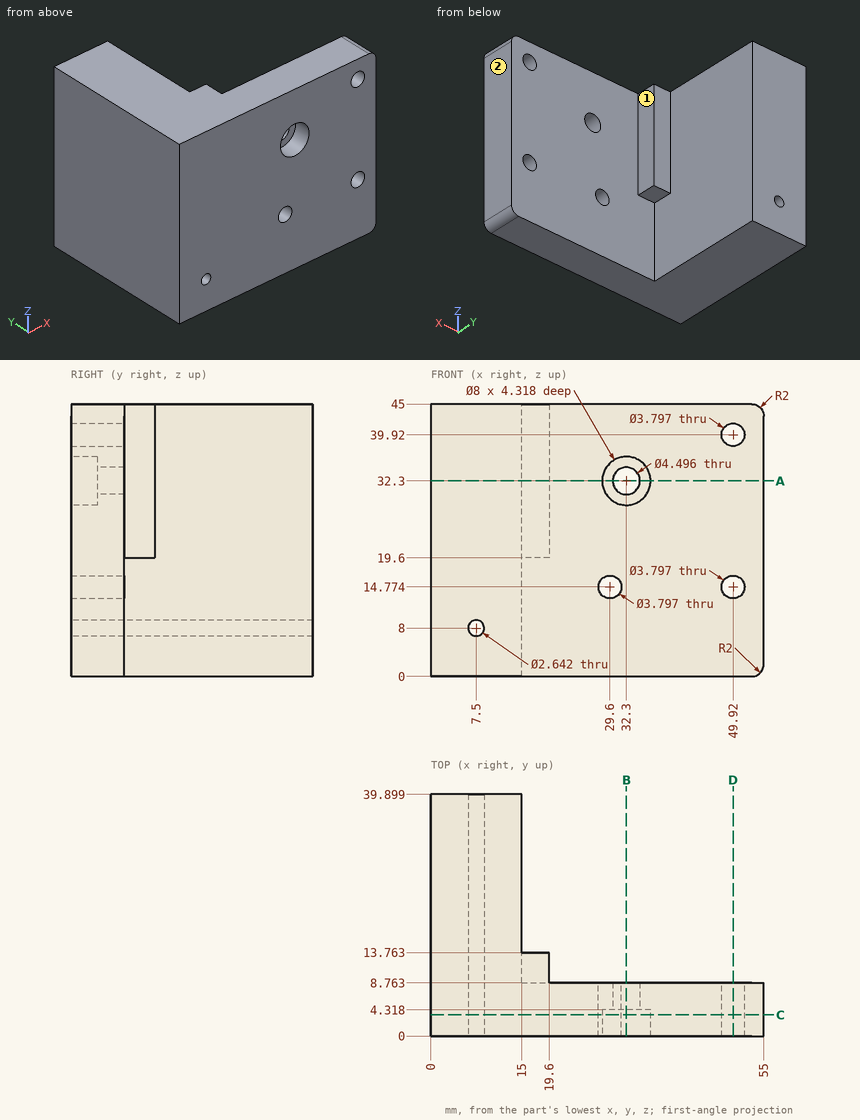
Print and shaded views of the part. All mm, measured from the part's lowest x, y and z. A direction names the side the tool comes from. Give positions to 0.01 mm unless a question says otherwise; leave off trailing zeros. Loops run counter-clockwise (first coordinate to the right, second up) from the corner with the lowest first, then second, coordinate; pieces in that order, holes last. Notation, with made-up numbers: (48.25, 9.25) -> (72.25, 9.25) arc R16 ccw to (72.25, 16.25) -> close; hole circle Ø2 at (55.25, 26). An arc over 180 degrees is marked (long way). One line per question, with ' | ' between items. Start each with the question number.
1) Pin check, flat tips, straight feed: pin 1 (2.5 mm diameter, centred on y = 12, z = 29.5, fed in from +X); pin 2 (6.5 mm diameter, centred on x = 32, z = 32.5, fed in from -Y); pin 3 (1 mm diameter, centred on y = 9.5, z = 13, fed in from +X). Stop position of each tip, or through.
2) Cut at C-C (y = 3.5). Give the cut face in (x, z).
3) Cut at D-D (x = 49.92). Give the cut face in (y, z), plus the area to 3 significant figures.
4) 3-axis set-ups, long thin cutter, end or side, ignore diameter. For the marked faces 1 and 2: which of +Z, -Z, +X, -X, +Y, -Y reach the whole face in a straight line?
5) Cut at A-A (z = 32.3). Give the cut face in (x, y).
6) Cut at B-B (x = 32.3). Give the cut face in (y, z), plus the area to 3 significant figures.
7) Probe L1, parallel to Z at x = 49.92, y = 3.5; L2, parallel to Z at x = 29.6, y = 4; L3, parallel to Z at x = 29.6, y = 5. List the from-to ranges inside material, lowest first.
Return value:
1) pin 1: x = 19.6 | pin 2: y = 4.32 | pin 3: x = 15
2) outline: (0, 0) -> (53, 0) arc R2 ccw to (55, 2) -> (55, 43) arc R2 ccw to (53, 45) -> (0, 45) -> close; hole circle Ø2.64 at (7.5, 8); hole circle Ø3.8 at (29.6, 14.77); hole circle Ø8 at (32.3, 32.3); hole circle Ø3.8 at (49.92, 14.77); hole circle Ø3.8 at (49.92, 39.92)
3) outline: (0, 0) -> (8.76, 0) -> (8.76, 12.88) -> (0, 12.88) -> close; (0, 16.67) -> (8.76, 16.67) -> (8.76, 38.02) -> (0, 38.02) -> close; (0, 41.82) -> (8.76, 41.82) -> (8.76, 45) -> (0, 45) -> close | area: 328 mm^2
4) face 1: +Z, -Z, +X, +Y | face 2: +Z, -Z, +X, +Y, -Y
5) outline: (0, 0) -> (28.3, 0) -> (28.3, 4.32) -> (30.05, 4.32) -> (30.05, 8.76) -> (19.6, 8.76) -> (19.6, 13.76) -> (15, 13.76) -> (15, 39.9) -> (0, 39.9) -> close; (34.55, 4.32) -> (36.3, 4.32) -> (36.3, 0) -> (55, 0) -> (55, 8.76) -> (34.55, 8.76) -> close
6) outline: (0, 0) -> (8.76, 0) -> (8.76, 30.05) -> (4.32, 30.05) -> (4.32, 28.3) -> (0, 28.3) -> close; (0, 36.3) -> (4.32, 36.3) -> (4.32, 34.55) -> (8.76, 34.55) -> (8.76, 45) -> (0, 45) -> close | area: 340 mm^2
7) L1: 0 to 12.88, 16.67 to 38.02, 41.82 to 45 | L2: 0 to 12.88, 16.67 to 29.35, 35.25 to 45 | L3: 0 to 12.88, 16.67 to 45
